Geometry: final body of the model. Coordinates: model frame, mm. Face numbers are marked on the shaded views. A direction names the side the tool comes from. Round coordinates to 2 decimals unless told otherwise and drop trailing zeros. Order: outer loops, then holes, each group sorted by start corner. A loop starts at its lowest first (then second) coordinate and runs counter-clockwise, first axis right, second up. Notation, with made-up numbers: M 77.5,45.5 L 88.5,45.5 A17 cw 88.5,74.5 Z; hole C 48,74 d9. An arc over 180 degrees is marked long. Return JSON: item names as keys, results as strings. Group by question number.
Q1. Cut plane B-B on z = 12. Output: boundary loops of the cut face in (x, y), and give its area (4 significant figures).
Q2. Cut plane C-C on y = 39.95. Count the separate pieces of the cut face and the enclosed holes in it, and give its area (3 significant figures).
Q3. Access query for the marked faces 1, 2 and 3. Directions: +Z, -Z, +X, -X, +Y, -Y. A direction counts if a zero-diameter tool reaches every point of the face in a straight line with its end or side. Return the directions, or none.
Q4. Cut plane A-A on x = -6.5. Output: boundary loops of the cut face in (y, z).
Q5. Ray query, probe 1 along X at (y, z) = (-39.95, 5.85); probe 2 along Y at (x, z) = (-15, 6.95); probe 3 along Y at (x, z) = (26, 2.25). Return the intervals inside material, ascending.
Q6. Contact query for flat-ended pins moving along their axis: pin 1 (3 mm diameter, centred on x = -13.5, y = 14.5, fed in from -Z); pin 2 (5 mm diameter, centred on x = -13, y = 7.5, fed in from +Z). Output: stop coordinate, or through.
Q7. Cut plane D-D on y = -7.5. Output: boundary loops of the cut face in (x, z).
Q8. Mould query, pull axis X, two halves, no side actions, for the marked faces 4, 5 and 6. Classes: released by +X, released by -X, zero draft, split by the parting line, or undercut.
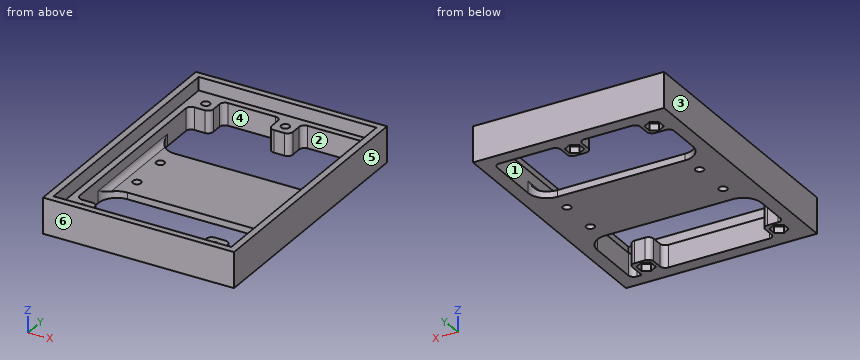
```python
from build123d import *

# Parameters (mm, degrees)
ESQUISSE1_W             = 72
ESQUISSE1_H             = 97.9
ESQUISSE1_R             = 1.55
BOSS_EXTRU_1_DEPTH      = 8.4
ENL_V_MAT_EXTRU_1_DEPTH = 2.5
ESQUISSE3_W             = 72
ESQUISSE3_H             = 97.9
ESQUISSE3_W_2           = 67
ESQUISSE3_H_2           = 92.9
BOSS_EXTRU_2_DEPTH      = 5
ESQUISSE4_W             = 72
ESQUISSE4_H             = 30.283908022
ESQUISSE4_R             = 1.55
BOSS_EXTRU_3_DEPTH      = 2.5
CONG_2_R                = 7
CONG_4_R                = 2


with BuildPart() as part:
    # Esquisse1 → Boss.-Extru.1 (new body)
    with BuildSketch(Plane.XY):
        with Locations((12, 0)):
            Rectangle(ESQUISSE1_W, ESQUISSE1_H)
        with Locations((15, 39.95)):
            Circle(ESQUISSE1_R, mode=Mode.SUBTRACT)
        with Locations((-15, 39.95)):
            Circle(ESQUISSE1_R, mode=Mode.SUBTRACT)
        with Locations((-15, -39.95)):
            Circle(ESQUISSE1_R, mode=Mode.SUBTRACT)
        with Locations((35.1, -39.95)):
            Circle(ESQUISSE1_R, mode=Mode.SUBTRACT)
        Polygon((-19, 35.95), (-11, 35.95), (-11, 43.95), (11, 43.95), (11, 35.95), (19, 35.95), (19, 43.95), (43, 43.95), (43, -43.95), (39.1, -43.95), (39.1, -35.95), (31.1, -35.95), (31.1, -43.95), (-11, -43.95), (-11, -35.95), (-19, -35.95), align=None, mode=Mode.SUBTRACT)
    extrude(amount=BOSS_EXTRU_1_DEPTH)

    # Esquisse2 → Enlèv. mat.-Extru.1 (cut)
    with BuildSketch(Plane(origin=(0, 0, 0), x_dir=(-1, 0, 0), z_dir=(0, 0, -1))):
        Polygon((-15, 36.774573519), (-12.25, 38.36228676), (-12.25, 41.53771324), (-15, 43.125426481), (-17.75, 41.53771324), (-17.75, 38.36228676), align=None)
        Polygon((14.996275716, 36.774575703), (17.748135966, 38.359062527), (17.751860251, 41.534486823), (15.003724284, 43.125424297), (12.251864034, 41.540937473), (12.248139749, 38.365513177), align=None)
        Polygon((15, -43.125426481), (17.75, -41.53771324), (17.75, -38.36228676), (15, -36.774573519), (12.25, -38.36228676), (12.25, -41.53771324), align=None)
        Polygon((-35.1, -43.125426481), (-32.35, -41.53771324), (-32.35, -38.36228676), (-35.1, -36.774573519), (-37.85, -38.36228676), (-37.85, -41.53771324), align=None)
    extrude(amount=-ENL_V_MAT_EXTRU_1_DEPTH, mode=Mode.SUBTRACT)

    # Esquisse3 → Boss.-Extru.2 (add)
    with BuildSketch(Plane.XY.offset(8.4)):
        with Locations((12, 0)):
            Rectangle(ESQUISSE3_W, ESQUISSE3_H)
        with Locations((12, 0)):
            Rectangle(ESQUISSE3_W_2, ESQUISSE3_H_2, mode=Mode.SUBTRACT)
    extrude(amount=BOSS_EXTRU_2_DEPTH)

    # Esquisse4 → Boss.-Extru.3 (add)
    with BuildSketch(Plane(origin=(0, 0, 0), x_dir=(-1, 0, 0), z_dir=(0, 0, -1))):
        with Locations((-12, 0)):
            Rectangle(ESQUISSE4_W, ESQUISSE4_H)
        with Locations((-37, 7.5)):
            Circle(ESQUISSE4_R, mode=Mode.SUBTRACT)
        with Locations((-37, -7.5)):
            Circle(ESQUISSE4_R, mode=Mode.SUBTRACT)
        with Locations((13, -7.5)):
            Circle(ESQUISSE4_R, mode=Mode.SUBTRACT)
        with Locations((13, 7.5)):
            Circle(ESQUISSE4_R, mode=Mode.SUBTRACT)
    extrude(amount=-BOSS_EXTRU_3_DEPTH)

    # Congé2
    cong_2_edges = [part.edges().sort_by_distance(p)[0] for p in [
        (43, -15.141954011, 1.25),
        (43, 15.141954011, 1.25),
        (-19, 15.141954011, 1.25),
        (-19, -15.141954011, 1.25),
    ]]
    fillet(cong_2_edges, radius=CONG_2_R)

    # Congé4
    cong_4_edges = [part.edges().sort_by_distance(p)[0] for p in [
        (43, 0, 2.5),
        (-19, 0, 2.5),
        (-19, 35.95, 4.2),
        (-19, -35.95, 4.2),
        (-11, -35.95, 4.2),
        (-11, -43.95, 4.2),
        (31.1, -43.95, 4.2),
        (31.1, -35.95, 4.2),
        (39.1, -35.95, 4.2),
        (43, -43.95, 4.2),
        (43, 43.95, 4.2),
        (19, 43.95, 4.2),
        (19, 35.95, 4.2),
        (11, 35.95, 4.2),
        (11, 43.95, 4.2),
        (-11, 43.95, 4.2),
        (-11, 35.95, 4.2),
    ]]
    fillet(cong_4_edges, radius=CONG_4_R)


solid = part.part
```
Result sheet:
{
 "1": {"outline": "M -24,-48.95 L 48,-48.95 L 48,48.95 L -24,48.95 Z; hole M -21.5,-46.45 L 45.5,-46.45 L 45.5,46.45 L -21.5,46.45 Z", "area": "824.5 mm²"},
 "2": {"separate pieces": "5", "enclosed holes": "0", "area": "179 mm²"},
 "3": {"face 1": "+Z", "face 2": "+Z, -Z", "face 3": "+Z, -Z, -X, +Y, -Y"},
 "4": {"outline": "M -48.95,0 L -43.95,0 L -43.95,8.4 L -46.45,8.4 L -46.45,13.4 L -48.95,13.4 Z; M -15.14,0 L 15.14,0 L 15.14,2.5 L -15.14,2.5 Z; M 43.95,0 L 48.95,0 L 48.95,13.4 L 46.45,13.4 L 46.45,8.4 L 43.95,8.4 Z"},
 "5": {"probe 1": "x = -24 to -16.55, -13.45 to -11, 31.1 to 33.55, 36.65 to 39.1, 43 to 48", "probe 2": "y = -48.95 to -41.5, -38.4 to -35.95, 35.95 to 38.4, 41.5 to 48.95", "probe 3": "y = -48.95 to -43.95, -15.14 to 15.14, 43.95 to 48.95"},
 "6": {"pin 1": "stops at z = 0", "pin 2": "stops at z = 2.5"},
 "7": {"outline": "M -24,0 L -14.55,0 L -14.55,2.5 L -17,2.5 A2 cw -19,4.5 L -19,8.4 L -21.5,8.4 L -21.5,13.4 L -24,13.4 Z; M -11.45,0 L 35.45,0 L 35.45,2.5 L -11.45,2.5 Z; M 38.55,0 L 48,0 L 48,13.4 L 45.5,13.4 L 45.5,8.4 L 43,8.4 L 43,4.5 A2 cw 41,2.5 L 38.55,2.5 Z"},
 "8": {"face 4": "undercut", "face 5": "released by +X", "face 6": "zero draft"}
}
